Could you check a few things on this drawing? It's one solid part, dimensions in mm from its lowest x, y, z. A direction names the side the tool comes from. Give positions to 0.01 mm unless a question says otherwise; leave off trailing zeros. Write each loop counter-clockwise with the first axis right and the second up, starting at its lowest first coordinate (ties: lowest second). Pieces come first, ordered by that corner, then holes. Notation, with made-up numbers: (12, -14.75) -> (43, -14.75) arc R18 cw to (43, 19.25) -> close; hole circle Ø11 at (71.25, -7). An arc over 180 degrees is marked (long way). Use CSV: the item, a comma, the result in double quotes. Start each with the question number.
(1) Suppose I cut it at A-A on x = 7. List the corners of the cut face in (y, z) for me, plus the area to 3 significant figures.
(2) Suppose I cut it at C-C on z = 9.25. List the corners of the cut face in (x, y) for me.
(3) Suppose I cut it at B-B on z = 5. List the corners of the cut face in (x, y) for me.
(4) Which directions (+Z, -Z, +X, -X, +Y, -Y) give clear straight access to the entire face, cutting with the end or side of a thin tool? Please do the marked faces 4 and 5.
(5) For pin 1 Ø4 at (y, z) = (12, 8.5) entering from +X, with a flat end and sliding along its axis, tell me the tip position at first contact or that it passes through.
(6) Suppose I cut it at D-D on y = 11. List the corners of the cut face in (x, z) for me, plus the area to 3 significant figures.
(7) I need wall thicknesses on L1, parallel to X at y = 16.9, z = 5; L2, parallel to Z at x = 4.5, y = 15.75; L3, parallel to Y at x = 5, z = 9.5. Which ranges of each line are inside material? Lowest first, please. Write a range as [from, to].
(8) If we mould it in two halves opening along Z, with no side actions, what happens to the marked faces 1, 2 and 3? For each: pulls with the +Z half, pulls with the -Z half, needs draft (parallel to the pull), parting line crosses it, or undercut.
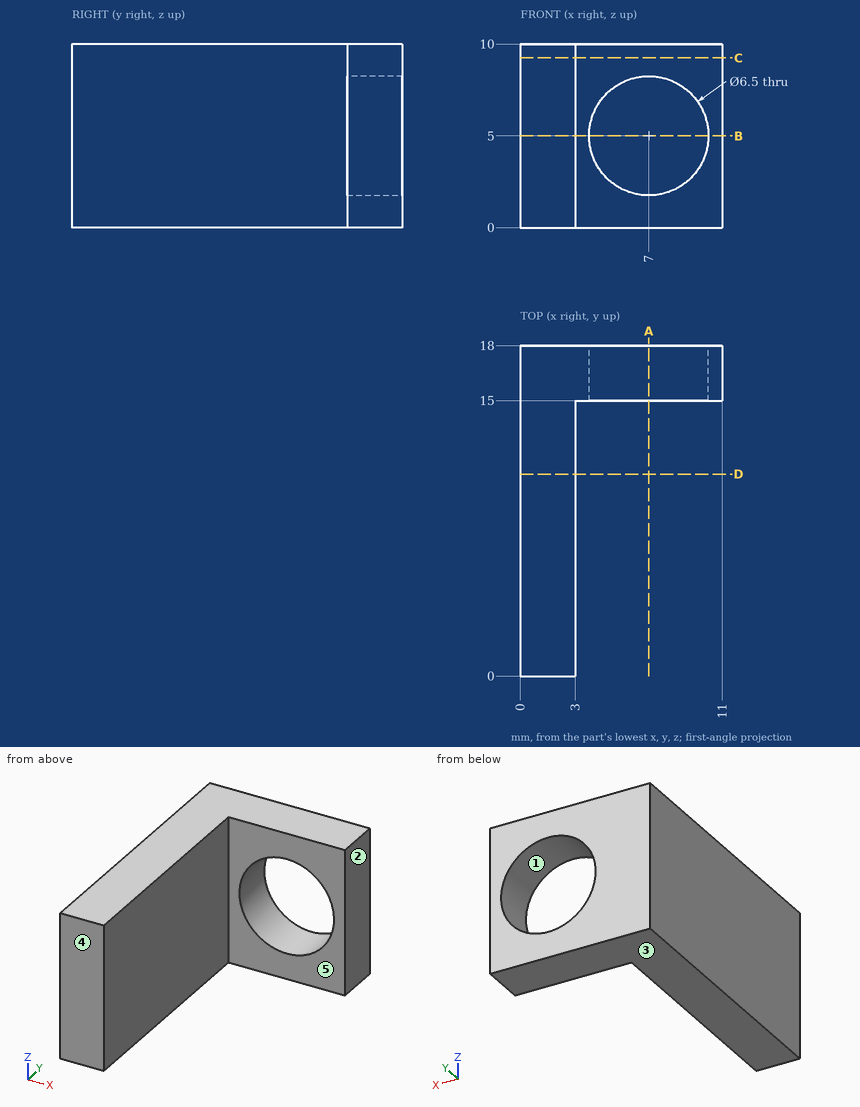
Geometry says:
1,outline,"(15, 0) -> (18, 0) -> (18, 1.75) -> (15, 1.75) -> close; (15, 8.25) -> (18, 8.25) -> (18, 10) -> (15, 10) -> close"
1,area,"10.5 mm²"
2,outline,"(0, 0) -> (3, 0) -> (3, 15) -> (11, 15) -> (11, 18) -> (0, 18) -> close"
3,outline,"(0, 0) -> (3, 0) -> (3, 15) -> (3.75, 15) -> (3.75, 18) -> (0, 18) -> close; (10.25, 15) -> (11, 15) -> (11, 18) -> (10.25, 18) -> close"
4,face 4,"+Z, -Z, +X, -X, -Y"
4,face 5,"+Z, -Z, +X, -Y"
5,pin 1,"x = 3"
6,outline,"(0, 0) -> (3, 0) -> (3, 10) -> (0, 10) -> close"
6,area,"30.0 mm²"
7,L1,"[0, 3.75], [10.25, 11]"
7,L2,"[0, 2.92], [7.08, 10]"
7,L3,"[15, 18]"
8,face 1,"undercut"
8,face 2,"needs draft"
8,face 3,"pulls with the -Z half"
